from build123d import *

# Parameters (mm, degrees)
SKETCH1_W                        = 73
SKETCH1_H                        = 73
SKETCH1_R                        = 3.2
SKETCH1_R_2                      = 22.5
BOSS_EXTRUDE1_DEPTH              = 6
TAP_DRILL_FOR_M6_HELICOIL1_D     = 6.25
TAP_DRILL_FOR_M6_HELICOIL1_DEPTH = 11.94
TAP_DRILL_FOR_M6_HELICOIL1_TIP   = 1.877689434


with BuildPart() as part:
    # Sketch1 → Boss-Extrude1 (new body)
    with BuildSketch(Plane(origin=(0, 0, 0), x_dir=(1, 0, 0), z_dir=(0, 1, 0))):
        with Locations((36.5, 36.5)):
            Rectangle(SKETCH1_W, SKETCH1_H)
        with Locations(Location((36.5, 64, 0), (0, 0, 270))):
            Circle(SKETCH1_R, mode=Mode.SUBTRACT)
        with Locations(Location((63.582213208, 31.724675114, 0), (0, 0, 270))):
            Circle(SKETCH1_R, mode=Mode.SUBTRACT)
        with Locations(Location((9.417786792, 31.724675114, 0), (0, 0, 270))):
            Circle(SKETCH1_R, mode=Mode.SUBTRACT)
        with Locations(Location((36.5, 36.5, 0), (0, 0, 270))):
            Circle(SKETCH1_R_2, mode=Mode.SUBTRACT)
    extrude(amount=BOSS_EXTRUDE1_DEPTH)

    # Tap Drill for M6 Helicoil1
    with Locations(Plane(origin=(0, 0, 0), x_dir=(-1, 0, 0), z_dir=(0, -1, 0))):
        with Locations((-11.5, 11.5), (-61.5, 11.5), (-61.5, 61.5)):
            Hole(TAP_DRILL_FOR_M6_HELICOIL1_D / 2, depth=TAP_DRILL_FOR_M6_HELICOIL1_DEPTH)
            with Locations((0, 0, -(TAP_DRILL_FOR_M6_HELICOIL1_DEPTH + TAP_DRILL_FOR_M6_HELICOIL1_TIP / 2))):  # 118° drill point
                Cone(0, TAP_DRILL_FOR_M6_HELICOIL1_D / 2, TAP_DRILL_FOR_M6_HELICOIL1_TIP, mode=Mode.SUBTRACT)


solid = part.part
Read the model definition and answer for the solid it produces. Units are mm, in the model's axes. Give positions to 0.01 mm unless a question says otherwise; leave off trailing zeros. Loops run counter-clockwise (first coordinate to the right, second up) from the corner with the lowest first, then second, coordinate; pieces in that order, holes last. Notation, with made-up numbers: (70.5, 70) -> (107.5, 70) arc R25 ccw to (107.5, 98) -> close; hole circle Ø3 at (48.25, 77.5). An arc over 180 degrees is marked (long way). Use a Markdown table: item, result.
Q1. Section A-A, the plane z = -11.5 is taken. Determine the outline of the cut face in (x, y) (3 decimals), then the cut area to 3 significant figures.
Solved:
| item | result |
|---|---|
| outline | (0, 0) -> (8.375, 0) -> (8.375, 6) -> (0, 6) -> close; (14.625, 0) -> (58.375, 0) -> (58.375, 6) -> (14.625, 6) -> close; (64.625, 0) -> (73, 0) -> (73, 6) -> (64.625, 6) -> close |
| area | 363 mm^2 |
Q2. Find the intervals of material crossed by line 1 along X through (y, z) = (2.75, -64) (3 decimals); line 2 along X through (y, z) = (2.5, -61.5) (1 decimal); line 3 along Z through (x, y) = (37.5, 3.8), in increasing order.
Solved:
| item | result |
|---|---|
| line 1 | x = 0 to 33.3, 39.7 to 59.625, 63.375 to 73 |
| line 2 | x = 0 to 34.5, 38.5 to 58.4, 64.6 to 73 |
| line 3 | z = -73 to -67.04, -60.96 to -58.98, -14.02 to 0 |
Q3. Section B-B, the plane z = -36.5 is taken. Determine the outline of the cut face in (x, y).
Solved:
| item | result |
|---|---|
| outline | (0, 0) -> (14, 0) -> (14, 6) -> (0, 6) -> close; (59, 0) -> (73, 0) -> (73, 6) -> (59, 6) -> close |
Q4. Section C-C, the plane x = 36.5 is taken. Determine the outline of the cut face in (y, z).
Solved:
| item | result |
|---|---|
| outline | (0, -73) -> (6, -73) -> (6, -67.2) -> (0, -67.2) -> close; (0, -60.8) -> (6, -60.8) -> (6, -59) -> (0, -59) -> close; (0, -14) -> (6, -14) -> (6, 0) -> (0, 0) -> close |
Q5. Section D-D, the plane x = 21 is taken. Determine the outline of the cut face in (y, z).
Solved:
| item | result |
|---|---|
| outline | (0, -73) -> (6, -73) -> (6, -52.81) -> (0, -52.81) -> close; (0, -20.19) -> (6, -20.19) -> (6, 0) -> (0, 0) -> close |
Q6. Determine the mould class of faces 1 (the face through (64.48, 3.04, -62.44)), 2 (the face through (73, 3, -36)), 3 (the face through (20, 0, -53)), 4 (the face through (39, 3, -66)) for opening direction X: pulls with the +X half, pulls with the -X half, needs draft (parallel to the pull), parting line crosses it, or undercut.
Solved:
| item | result |
|---|---|
| face 1 | undercut |
| face 2 | pulls with the +X half |
| face 3 | needs draft |
| face 4 | undercut |
Q7. This flat-tipped pin is pushed along its axis until it touches: pin 1 (2 mm diameter, centred on x = 45.5, y = 1, fed in from +Z). Where does it stop, or does it pass through?
Solved:
| item | result |
|---|---|
| pin 1 | stops at z = 0 |
